Here's the drawing with two shaded views (mm, measured from the low corner). I have some questions. A direction names the side the tool comes from. Give positions to 0.01 mm unless a question says otherwise; leave off trailing zeros. Order: outer loops, then holes, each group sorted by start corner. A loop starts at its lowest first (then second) coordinate and runs counter-clockwise, first axis right, second up. Notation, with made-up numbers: M 65.25,69.25 L 122.25,69.25 A30 cw 122.25,93.25 Z; hole C 60.25,-17.75 d6. An arc over 180 degrees is marked long. Write each question's results on one line, items separated by ' | '.
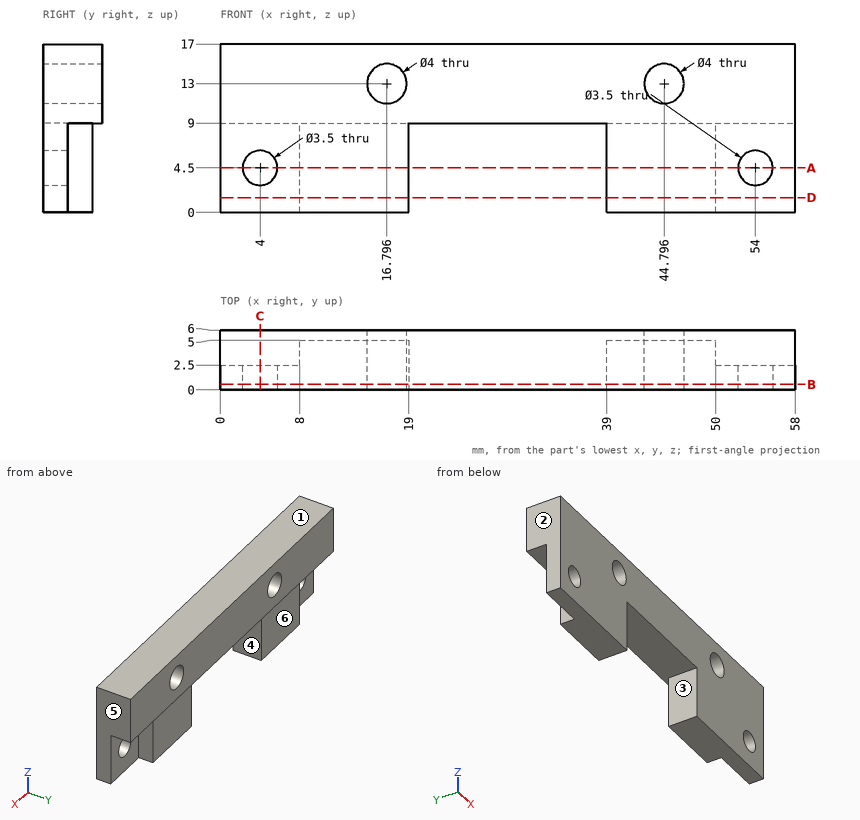
(1) Imagine slicing it at B-B, the plane y = 0.55. Write out the boundary of the cut face in (x, z).
Data:
outline: M 0,0 L 19,0 L 19,9 L 39,9 L 39,0 L 58,0 L 58,17 L 0,17 Z; hole C 4,4.5 d3.5; hole C 16.8,13 d4; hole C 44.8,13 d4; hole C 54,4.5 d3.5
(2) We'd pull the mould along X, two halves only. Please class the marked faces 1, 2 and 3: +X half, -X half, draft (parallel to the pull), parting line (faces both ways), or undercut.
Data:
face 1: draft | face 2: -X half | face 3: undercut
(3) Will these pins go through, and if not, where does the flat tip stop? P1, Ø3, axis at x = 44.8, z = 13, coming from the -Y side; P2, Ø1.2, axis at y = 4.5, z = 4.5, coming from the -X side; P3, Ø1.8, axis at x = 21, y = 2, coming from the -Z side; P4, Ø4, axis at x = 5.5, z = 5, coming from the +Y side.
Data:
P1: passes through | P2: stops at x = 8 | P3: stops at z = 9 | P4: stops at y = 2.5
(4) For the marked faces 4, 5 and 6, which set-ups out of +Z, -Z, +X, -X, +Y, -Y let a thin tool reach every point of the face, with its end or its side?
Data:
face 4: -Z, +Y, -Y | face 5: +Z, -Z, +X, +Y, -Y | face 6: -Z, +X, -X, +Y
(5) I need wall thicknesses on L1, parallel to X at y = 1.45, z = 4.75; L2, parallel to Z at x = 4, y = 0.75; L3, parallel to Y at x = 16.5, z = 5.25. Which ranges of each line are inside material? Lowest first, please. Write a range as from..to.
Data:
L1: x = 0..2.27, 5.73..19, 39..52.27, 55.73..58 | L2: z = 0..2.75, 6.25..17 | L3: y = 0..5
(6) Imagine slicing it at A-A, the plane z = 4.5. Write out the boundary of the cut face in (x, y).
Data:
outline: M 0,0 L 2.25,0 L 2.25,2.5 L 0,2.5 Z; M 5.75,0 L 19,0 L 19,5 L 8,5 L 8,2.5 L 5.75,2.5 Z; M 39,0 L 52.25,0 L 52.25,2.5 L 50,2.5 L 50,5 L 39,5 Z; M 55.75,0 L 58,0 L 58,2.5 L 55.75,2.5 Z
(7) Imagine slicing it at D-D, the plane z = 1.5. Write out the boundary of the cut face in (x, y), plus the area to 3 significant figures.
Data:
outline: M 0,0 L 19,0 L 19,5 L 8,5 L 8,2.5 L 0,2.5 Z; M 39,0 L 58,0 L 58,2.5 L 50,2.5 L 50,5 L 39,5 Z | area: 150 mm2
(8) Imagine slicing it at C-C, the plane x = 4. Write out the boundary of the cut face in (y, z).
Data:
outline: M 0,0 L 2.5,0 L 2.5,2.75 L 0,2.75 Z; M 0,6.25 L 2.5,6.25 L 2.5,9 L 6,9 L 6,17 L 0,17 Z
